Read the model definition and answer for the solid it produces. Units are mm, in the model's axes. Face numbers are marked on the shaded views. A direction names the side the tool comes from. Coordinates: 2 decimals unless noted, no trailing zeros. Loops run counter-clockwise (first coordinate to the right, second up) from the corner with the lowest first, then second, coordinate; pieces in that order, holes last.
Q1. Which of the six approach directions +Z, -Z, +X, -X, +Y, -Y give full straight-line access (tool end or side, diameter ignored) to the marked faces 1, 2, 3 and 4?
Q2. Section A-A (y = 9) is taken. Give the vertices of the cut face in (x, z).
Q3. Flat-ended cylindrical pins translate along their axes: P1, Ø2, axis at x = -27, z = 4, coming from the -Y side; P2, Ø6, axis at y = -18.5, z = 12.5, coming from the -X side; P3, Ø9.5, axis at y = -4, z = 6, coming from the +X side. Find the tip coordinate at first contact, or state that the pin passes through.
Q4. Straight lines are drawn through the part: line 1 (Y direction, x = -6.5, z = 8); line 2 (Y direction, x = -15, z = 14). For each, find the intervals that lie inside material, in ascending order.
Q5. Section C-C (x = -10) is taken. Give the vertices of the cut face in (y, z).
Q6. The mould has two halves that part along X. Classify the marked faces 5, 6 and 7: pulls with the +X half, pulls with the -X half, needs draft (parallel to the pull), parting line crosses it, or undercut.
Q7. Section D-D (z = 9) is taken. Give the vertices of the cut face in (x, y).
Q8. Section B-B (z = 4) is taken. Count the separate pieces of the cut face and the enclosed holes in it, then the cut area to 3 significant figures.
from build123d import *

# Parameters (mm, degrees)
PAD_DEPTH       = 15
PAD_DEPTH_BACK  = 1.5
POCKET_DEPTH    = 2.5
POCKET001_DEPTH = 12
SKETCH003_W     = 9.5
SKETCH003_H     = 13.5
POCKET002_DEPTH = 7
SKETCH004_W     = 7
SKETCH004_H     = 4
POCKET003_DEPTH = 7
SKETCH006_W     = 7
SKETCH006_H     = 4
SKETCH006_W_2   = 9
POCKET004_DEPTH = 7
SKETCH007_W     = 66
SKETCH007_H     = 66
POCKET005_DEPTH = 15


with BuildPart() as part:
    # Sketch → Pad (new body, two sides)
    with BuildSketch(Plane.XY) as pad_sk:
        with BuildLine():
            Line((-32, 33), (32, 33))
            ThreePointArc((33, 32), (32.707107, 32.707107), (32, 33))
            Line((33, 32), (33, -32))
            ThreePointArc((32, -33), (32.707107, -32.707107), (33, -32))
            Line((32, -33), (-32, -33))
            ThreePointArc((-33, -32), (-32.707107, -32.707107), (-32, -33))
            Line((-33, -32), (-33, 32))
            ThreePointArc((-32, 33), (-32.707107, 32.707107), (-33, 32))
        make_face()
    extrude(amount=PAD_DEPTH)
    extrude(pad_sk.sketch, amount=-PAD_DEPTH_BACK)

    # Sketch001 (on Face10 of Pad) → Pocket (cut)
    with BuildSketch(Plane.XY.offset(15)):
        with BuildLine():
            Line((-26, 27), (26, 27))
            ThreePointArc((27, 26), (26.707107, 26.707107), (26, 27))
            Line((27, 26), (27, -26))
            ThreePointArc((26, -27), (26.707107, -26.707107), (27, -26))
            Line((26, -27), (-26, -27))
            ThreePointArc((-27, -26), (-26.707107, -26.707107), (-26, -27))
            Line((-27, -26), (-27, 26))
            ThreePointArc((-26, 27), (-26.707107, 26.707107), (-27, 26))
        make_face()
    extrude(amount=-POCKET_DEPTH, mode=Mode.SUBTRACT)

    # Sketch002 (on Face19 of Pocket) → Pocket001 (cut)
    with BuildSketch(Plane.XY.offset(12.5)):
        with BuildLine():
            Line((-25, 26), (25, 26))
            ThreePointArc((26, 25), (25.707107, 25.707107), (25, 26))
            Line((26, 25), (26, -25))
            ThreePointArc((25, -26), (25.707107, -25.707107), (26, -25))
            Line((25, -26), (-25, -26))
            ThreePointArc((-26, -25), (-25.707107, -25.707107), (-25, -26))
            Line((-26, -25), (-26, 25))
            ThreePointArc((-25, 26), (-25.707107, 25.707107), (-26, 25))
        make_face()
    extrude(amount=-POCKET001_DEPTH, mode=Mode.SUBTRACT)

    # Sketch003 (on Face1 of Pocket001) → Pocket002 (cut)
    with BuildSketch(Plane(origin=(-33, 0, 0), x_dir=(0, -1, 0), z_dir=(-1, 0, 0))):
        with Locations((18.04, 8.25)):
            Rectangle(SKETCH003_W, SKETCH003_H)
    extrude(amount=-POCKET002_DEPTH, mode=Mode.SUBTRACT)

    # Sketch004 (on Face1 of Pocket002) → Pocket003 (cut)
    with BuildSketch(Plane(origin=(-33, 0, 0), x_dir=(0, -1, 0), z_dir=(-1, 0, 0))):
        with Locations((-8.71, 3.5)):
            Rectangle(SKETCH004_W, SKETCH004_H)
    extrude(amount=-POCKET003_DEPTH, mode=Mode.SUBTRACT)

    # Sketch006 (on Face15 of Pocket003) → Pocket004 (cut)
    with BuildSketch(Plane.YZ.offset(33)):
        with Locations((-17, 3.5)):
            Rectangle(SKETCH006_W, SKETCH006_H)
        with Locations((10.8, 3.5)):
            Rectangle(SKETCH006_W_2, SKETCH006_H)
    extrude(amount=-POCKET004_DEPTH, mode=Mode.SUBTRACT)

    # Sketch007 (on Face5 of Pocket004) → Pocket005 (cut)
    with BuildSketch(Plane.XY.offset(15)):
        Rectangle(SKETCH007_W, SKETCH007_H)
        with BuildLine():
            Line((28, 26), (28, -26))
            ThreePointArc((26, -28), (27.414214, -27.414214), (28, -26))
            Line((26, -28), (-26, -28))
            ThreePointArc((-28, -26), (-27.414214, -27.414214), (-26, -28))
            Line((-28, -26), (-28, 26))
            ThreePointArc((-26, 28), (-27.414214, 27.414214), (-28, 26))
            Line((26, 28), (-26, 28))
            ThreePointArc((28, 26), (27.414214, 27.414214), (26, 28))
        make_face(mode=Mode.SUBTRACT)
    extrude(amount=-POCKET005_DEPTH, mode=Mode.SUBTRACT)


solid = part.part
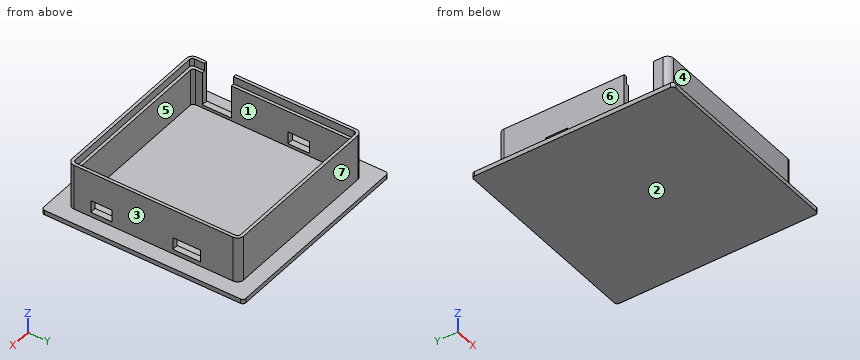
Numbers:
1. face 1: +Z
1. face 2: -Z, +X, -X, +Y, -Y
1. face 3: +Z, +X, +Y, -Y
1. face 4: +Z, +X, -X, -Y
2. outline: (-33, -1.5) - (33, -1.5) - (33, 0) - (28, 0) - (28, 1.5) - (26, 1.5) - (26, 0.5) - (-26, 0.5) - (-26, 1.5) - (-28, 1.5) - (-28, 0) - (-33, 0) - close; (-28, 5.5) - (-26, 5.5) - (-26, 12.5) - (-27, 12.5) - (-27, 15) - (-28, 15) - close; (26, 5.5) - (28, 5.5) - (28, 15) - (27, 15) - (27, 12.5) - (26, 12.5) - close
3. P1: stops at y = -28
3. P2: stops at x = 26
3. P3: stops at x = 28
4. line 1: y = -28 to -26, 26 to 28
4. line 2: y = -28 to -27, 27 to 28
5. outline: (-33, -1.5) - (33, -1.5) - (33, 0) - (28, 0) - (28, 15) - (27, 15) - (27, 12.5) - (26, 12.5) - (26, 0.5) - (-26, 0.5) - (-26, 12.5) - (-27, 12.5) - (-27, 15) - (-28, 15) - (-28, 0) - (-33, 0) - close
6. face 5: undercut
6. face 6: pulls with the -X half
6. face 7: needs draft
7. outline: (-28, -26) arc R2 ccw to (-26, -28) - (26, -28) arc R2 ccw to (28, -26) - (28, 26) arc R2 ccw to (26, 28) - (-26, 28) arc R2 ccw to (-28, 26) - (-28, -13.29) - (-26, -13.29) - (-26, 25) arc R1 cw to (-25, 26) - (25, 26) arc R1 cw to (26, 25) - (26, -25) arc R1 cw to (25, -26) - (-25, -26) arc R1 cw to (-26, -25) - (-26, -22.79) - (-28, -22.79) - close
8. separate pieces: 4
8. enclosed holes: 0
8. area: 364 mm2
